```python
from build123d import *

# Parameters (mm, degrees)
F0_W          = 30
F0_H          = 20
F0_R          = 2.5
F1_DEPTH      = 20
F1_DEPTH_BACK = 10


with BuildPart() as f1:
    # F0 (on Top) → F1 (new body, two sides)
    with BuildSketch(Plane.XY) as f1_sk:
        with Locations((-5.71409, -16.938188)):
            Rectangle(F0_W, F0_H)
        with Locations((-10.71409, -17.323306)):
            Circle(F0_R, mode=Mode.SUBTRACT)
    extrude(amount=F1_DEPTH)
    extrude(f1_sk.sketch, amount=-F1_DEPTH_BACK)


solid = f1.part
```
Here's how the part is built. I have some questions about the finished solid (model axes, mm). Coordinates: 2 decimals unless noted, no trailing zeros. Write each loop counter-clockwise with the first axis right and the second up, starting at its lowest first coordinate (ties: lowest second). Pieces come first, ordered by that corner, then holes. Notation, with made-up numbers: (55, 37.25) -> (93, 37.25) arc R22 ccw to (93, 58.25) -> close; hole circle Ø2 at (84, 35.5). An arc over 180 degrees is marked (long way). Use a Markdown table: item, result. Add a question column.
(1) If we section it at C-C, the plane z = 15.5: Write out the boundary of the cut face in (x, y), and give its area (3 significant figures).
(2) Please list where these lines run through material, in increasing order: line 1 (X direction, y = -17.5, z = 8.25); line 2 (X direction, y = -16.25, z = 11); line 3 (Y direction, x = -9, z = 3.5).
(3) I'm going to push a flat-ended pin straight in: P1, Ø3, axis at x = -10.71, y = -17.32, coming from the +Z side. Where does the tip first touch, or does it pass through?
(4) If we section it at B-B, the plane x = -10.25: Write out the boundary of the cut face in (y, z).
(5) We'd pull the mould along X, two halves only. Please class faces 1 (the flat face through (-6, -26.938, 5)), 2 (the cylindrical face through (-9.56, -19.54, 4.79)), 3 (the flat face through (9.286, -17, 5)): +X half, -X half, draft (parallel to the pull), parting line (faces both ways), or undercut.
(6) If we section it at A-A, the plane y = -19: Write out the boundary of the cut face in (x, z).
Outcome:
| question | item | result |
|---|---|---|
| 1 | outline | (-20.71, -26.94) -> (9.29, -26.94) -> (9.29, -6.94) -> (-20.71, -6.94) -> close; hole circle Ø5 at (-10.71, -17.32) |
| 1 | area | 580 mm^2 |
| 2 | line 1 | x = -20.71 to -13.21, -8.22 to 9.29 |
| 2 | line 2 | x = -20.71 to -12.97, -8.46 to 9.29 |
| 2 | line 3 | y = -26.94 to -19.14, -15.5 to -6.94 |
| 3 | P1 | passes through |
| 4 | outline | (-26.94, -10) -> (-19.78, -10) -> (-19.78, 20) -> (-26.94, 20) -> close; (-14.87, -10) -> (-6.94, -10) -> (-6.94, 20) -> (-14.87, 20) -> close |
| 5 | face 1 | draft |
| 5 | face 2 | undercut |
| 5 | face 3 | +X half |
| 6 | outline | (-20.71, -10) -> (-12.57, -10) -> (-12.57, 20) -> (-20.71, 20) -> close; (-8.86, -10) -> (9.29, -10) -> (9.29, 20) -> (-8.86, 20) -> close |
